from build123d import *

# Parameters (mm, degrees)
SKETCH1_W           = 107.763073452
SKETCH1_H           = 107.763073452
BOSS_EXTRUDE1_DEPTH = 3.175
CUT_EXTRUDE2_REACH  = 78.266
SKETCH4_R           = 50.8
FILLET1_R           = 6.35
CUT_EXTRUDE3_REACH  = 78.266
SKETCH5_R           = 2.665000004


with BuildPart() as part:
    # Sketch1 → Boss-Extrude1 (new body)
    with BuildSketch(Plane.XY):
        Rectangle(SKETCH1_W, SKETCH1_H)
    extrude(amount=BOSS_EXTRUDE1_DEPTH)

    # Sketch4 → Cut-Extrude2 (cut, up to next)
    with BuildSketch(Plane.XY.offset(3.175), mode=Mode.PRIVATE) as cut_extrude2_sk1:
        Circle(SKETCH4_R)
    cut_extrude2_tool1 = extrude(cut_extrude2_sk1.sketch, amount=-CUT_EXTRUDE2_REACH, mode=Mode.PRIVATE) & part.part
    add(cut_extrude2_tool1.solids().sort_by_distance((0, 0, 3.175))[0], mode=Mode.SUBTRACT)

    # Fillet1
    fillet1_edges = [part.edges().sort_by_distance(p)[0] for p in [
        (-53.881536726, -53.881536726, 1.5875),
        (-53.881536726, 53.881536726, 1.5875),
        (53.881536726, 53.881536726, 1.5875),
        (53.881536726, -53.881536726, 1.5875),
    ]]
    fillet(fillet1_edges, radius=FILLET1_R)

    # Sketch5 → Cut-Extrude3 (cut, up to next)
    with BuildSketch(Plane.XY.offset(3.175), mode=Mode.PRIVATE) as cut_extrude3_sk1:
        with Locations((-44.838745817, 44.838745817)):
            Circle(SKETCH5_R)
    cut_extrude3_tool1 = extrude(cut_extrude3_sk1.sketch, amount=-CUT_EXTRUDE3_REACH, mode=Mode.PRIVATE) & part.part
    # Sketch5 → Cut-Extrude3 (cut, up to next)
    with BuildSketch(Plane.XY.offset(3.175), mode=Mode.PRIVATE) as cut_extrude3_sk2:
        with Locations((44.963815393, 44.838745817)):
            Circle(SKETCH5_R)
    cut_extrude3_tool2 = extrude(cut_extrude3_sk2.sketch, amount=-CUT_EXTRUDE3_REACH, mode=Mode.PRIVATE) & part.part
    # Sketch5 → Cut-Extrude3 (cut, up to next)
    with BuildSketch(Plane.XY.offset(3.175), mode=Mode.PRIVATE) as cut_extrude3_sk3:
        with Locations((-44.838745817, -44.963815393)):
            Circle(SKETCH5_R)
    cut_extrude3_tool3 = extrude(cut_extrude3_sk3.sketch, amount=-CUT_EXTRUDE3_REACH, mode=Mode.PRIVATE) & part.part
    # Sketch5 → Cut-Extrude3 (cut, up to next)
    with BuildSketch(Plane.XY.offset(3.175), mode=Mode.PRIVATE) as cut_extrude3_sk4:
        with Locations((44.963815393, -44.963815393)):
            Circle(SKETCH5_R)
    cut_extrude3_tool4 = extrude(cut_extrude3_sk4.sketch, amount=-CUT_EXTRUDE3_REACH, mode=Mode.PRIVATE) & part.part
    add(cut_extrude3_tool1.solids().sort_by_distance((-44.838746, 44.838746, 3.175))[0], mode=Mode.SUBTRACT)
    add(cut_extrude3_tool2.solids().sort_by_distance((44.963815, 44.838746, 3.175))[0], mode=Mode.SUBTRACT)
    add(cut_extrude3_tool3.solids().sort_by_distance((-44.838746, -44.963815, 3.175))[0], mode=Mode.SUBTRACT)
    add(cut_extrude3_tool4.solids().sort_by_distance((44.963815, -44.963815, 3.175))[0], mode=Mode.SUBTRACT)


solid = part.part
Can you work these out from the model? Positions are in its coordinate system, mm. Give positions to 0.01 mm unless a question says otherwise; leave off trailing zeros. Order: outer loops, then holes, each group sorted by start corner. A loop starts at its lowest first (then second) coordinate and runs counter-clockwise, first axis right, second up. Notation, with made-up numbers: M 86,-1.75 L 96,-1.75 A10 ccw 96,14.25 Z; hole C 4,29 d5. An arc over 180 degrees is marked long. One line per item, written item: value.
Item 1: For pin 1 (5 mm diameter, centred on x = -44.84, y = 44.84, fed in from -Z), with a flat end and sliding along its axis, tell me the tip position at first contact or that it passes through.
Verdict:
pin 1: through
Item 2: Please list where these lines run through material, in increasing order: line 1 (Y direction, x = 0, z = 2); line 2 (X direction, y = 43.5, z = 2.5); line 3 (Y direction, x = 12.5, z = 1.85).
Verdict:
line 1: -53.88 to -50.8, 50.8 to 53.88
line 2: -53.88 to -47.14, -42.53 to -26.24, 26.24 to 42.66, 47.27 to 53.88
line 3: -53.88 to -49.24, 49.24 to 53.88
Item 3: If we section it at C-C on z = 1.15: Write out the boundary of the cut face in (x, y) (3 decimals), and give its area (3 significant figures).
Verdict:
outline: M -53.882,-47.532 A6.35 ccw -47.532,-53.882 L 47.532,-53.882 A6.35 ccw 53.882,-47.532 L 53.882,47.532 A6.35 ccw 47.532,53.882 L -47.532,53.882 A6.35 ccw -53.882,47.532 Z; hole C 0,0 d101.6; hole C -44.839,-44.964 d5.33; hole C -44.839,44.839 d5.33; hole C 44.964,-44.964 d5.33; hole C 44.964,44.839 d5.33
area: 3,380 mm2
Item 4: If we mould it in two halves opening along X, with no side actions, what happens to faces 1 (the face through (-52.07, 51.97, 1.61)), 2 (the face through (-40, 32, 0)), 3 (the face through (42.3, -44.85, 1.61))? For each: pulls with the +X half, pulls with the -X half, needs draft (parallel to the pull), parting line crosses it, or undercut.
Verdict:
face 1: pulls with the -X half
face 2: needs draft
face 3: undercut
Item 5: If we section it at A-A on y = 0: Write out the boundary of the cut face in (x, z) (3 decimals), and give its area (3 significant figures).
Verdict:
outline: M -53.882,0 L -50.8,0 L -50.8,3.175 L -53.882,3.175 Z; M 50.8,0 L 53.882,0 L 53.882,3.175 L 50.8,3.175 Z
area: 19.6 mm2
